CAD build for the part. Positions are in the model's coordinates, mm. A direction names the side the tool comes from. Round coordinates to 2 decimals unless told otherwise and drop trailing zeros. Loops run counter-clockwise (first coordinate to the right, second up) from the corner with the lowest first, then second, coordinate; pieces in that order, holes last. Notation, with made-up numbers: (42, 78.25) - (48, 78.25) arc R20 cw to (48, 86.25) - close; hole circle Ø9 at (10.5, -4.5). An arc over 180 degrees is marked (long way). One line per question, with ' | ' between items.
```python
from build123d import *

# Parameters (mm, degrees)
F2_DEPTH  = 16
F0_R      = 16
F3_DEPTH  = 25
F4_DEPTH  = 25
F6_DEPTH  = 1.5
F8_DEPTH  = 10
F10_DEPTH = 25
F11_R     = 0.75
F12_DEPTH = 8
F14_DEPTH = 25


with BuildPart() as f2:
    # F1 (on Front) → F2 (new body, symmetric)
    with BuildSketch(Plane.XZ):
        Polygon((16, 16), (0, 0), (16, 0), align=None)
    extrude(amount=F2_DEPTH, both=True)

    # F0 (on Top) → F3 (intersect)
    with BuildSketch(Plane.XY):
        Circle(F0_R)
    extrude(amount=F3_DEPTH, mode=Mode.INTERSECT)

    # F0 (on Top) → F4 (join)
    with BuildSketch(Plane.XY):
        Circle(F0_R)
    extrude(amount=-F4_DEPTH)

    # F5 (on face) → F6 (join)
    with BuildSketch(Plane(origin=(0, 0, 0), x_dir=(0, -1, 0), z_dir=(-0.707107, 0, 0.707107))):
        with BuildLine():
            Line((-0.184881, 0.507365), (0, 0))
            Line((0, 0), (0.54, 0))
            Line((0.54, 0), (13.54, 0))
            ThreePointArc((13.54, 0), (7.76415, 11.092771), (-4.635713, 12.721704))
            Line((-4.635713, 12.721704), (-0.184881, 0.507365))
        make_face()
    extrude(amount=F6_DEPTH)

    # F7 (on face) → F8 (join)
    with BuildSketch(Plane(origin=(0, 0, 0), x_dir=(0, -1, 0), z_dir=(-0.707107, 0, 0.707107))):
        Polygon((0, 0), (-0.184881, 0.507365), (-1.577233, 0), align=None)
    extrude(amount=F8_DEPTH)

    # F9 (on face) → F10 (cut)
    with BuildSketch(Plane.XY):
        with BuildLine():
            ThreePointArc((0, 16), (-16, 0), (0, -16))
            Line((0, -16), (0, 16))
        make_face()
    extrude(amount=F10_DEPTH, mode=Mode.SUBTRACT)

    # F11 (on face) → F12 (cut)
    with BuildSketch(Plane.XY):
        with Locations((-0.75, -0.54)):
            Circle(F11_R)
    extrude(amount=-F12_DEPTH, mode=Mode.SUBTRACT)

    # F13 (on face) → F14 (cut)
    with BuildSketch(Plane(origin=(0, 0, 0), x_dir=(0, -1, 0), z_dir=(-0.707107, 0, 0.707107))):
        with BuildLine():
            ThreePointArc((-16, 0), (0, 16), (16, 0))
            add(Edge.make_bspline(
                [(16, 0), (16, 22.627417), (0, 22.627417)],
                knots=[1.570796, 1.570796, 1.570796, 3.141593, 3.141593, 3.141593], degree=2, weights=[1, 0.707107, 1]))
            add(Edge.make_bspline(
                [(0, 22.627417), (-16, 22.627417), (-16, 0)],
                knots=[3.141593, 3.141593, 3.141593, 4.712389, 4.712389, 4.712389], degree=2, weights=[1, 0.707107, 1]))
        make_face()
    extrude(amount=-F14_DEPTH, mode=Mode.SUBTRACT)


solid = f2.part
```
(1) Two-plate mould, pull along Z, no slides. Class faces 4 (the face through (4.21, 2.44, 5.26)), 5 (the face through (-1, -1, -8)), 6 (the face through (0, 0, -25)), 7 (the face through (0, -6, 1)): released by +Z, released by -Z, zero draft, split by the parting line, or undercut.
Results found:
face 4: undercut | face 5: released by +Z | face 6: released by -Z | face 7: zero draft
(2) Tool access for faces 1 (the face through (7.25, -7.91, 8.29)), 2 (the face through (-6, 0, 0)), 3 (the face through (13.1, 0.35, 9.52)): list every direction of +Z, -Z, +X, -X, +Y, -Y with a clear straight run to the whole face (end or side of a thin tool).
Results found:
face 1: +Z | face 2: +Z, -X, +Y, -Y | face 3: +Z, +X
(3) Probe L1, parallel to Z at x = -2, y = -11; L2, parallel to Y at x = -0.75, z = -5.75; L3, parallel to X at y = -7.5, z = -16. List the from-to ranges inside material, lowest first.
Results found:
L1: z = -25 to 0 | L2: y = -15.98 to -1.29, 0.21 to 15.98 | L3: x = -14.13 to 14.13
(4) Cut at B-B, the plane x = -0.75. Write the cut outline in (y, z), then the cut area to 3 significant figures.
Results found:
outline: (-15.98, -25) - (15.98, -25) - (15.98, 0) - (0.21, 0) - (0.21, -8) - (-1.29, -8) - (-1.29, 0) - (-15.98, 0) - close | area: 787 mm²
(5) Cut at D-D, the plane z = -7. Write the cut outline in (x, y).
Results found:
outline: circle Ø32 at (0, 0); hole circle Ø1.5 at (-0.75, -0.54)
(6) Cut at C-C, the plane z = -11.5. Write the cut outline in (x, y).
Results found:
outline: circle Ø32 at (0, 0)
(7) Drop flat-ended pins along their axis: P1, Ø1.7, axis at x = -0.75, y = -0.54, coming from the +Z side; P2, Ø2, axis at x = 6.5, z = -11, coming from the +Y side (3 decimals); P3, Ø17.5, axis at x = -6.5, y = 3.5, coming from the +Z side. Give the stop position or say it passes through.
Results found:
P1: stops at z = 2.22 | P2: stops at y = 15.025 | P3: stops at z = 4.16
(8) Cut at A-A, the plane y = -7. Write the cut outline in (x, z).
Results found:
outline: (-14.39, -25) - (14.39, -25) - (14.39, 5.96) - (10.17, 10.17) - (8.2, 8.2) - (7.13, 9.26) - (0, 2.12) - (0, 0) - (-14.39, 0) - close
